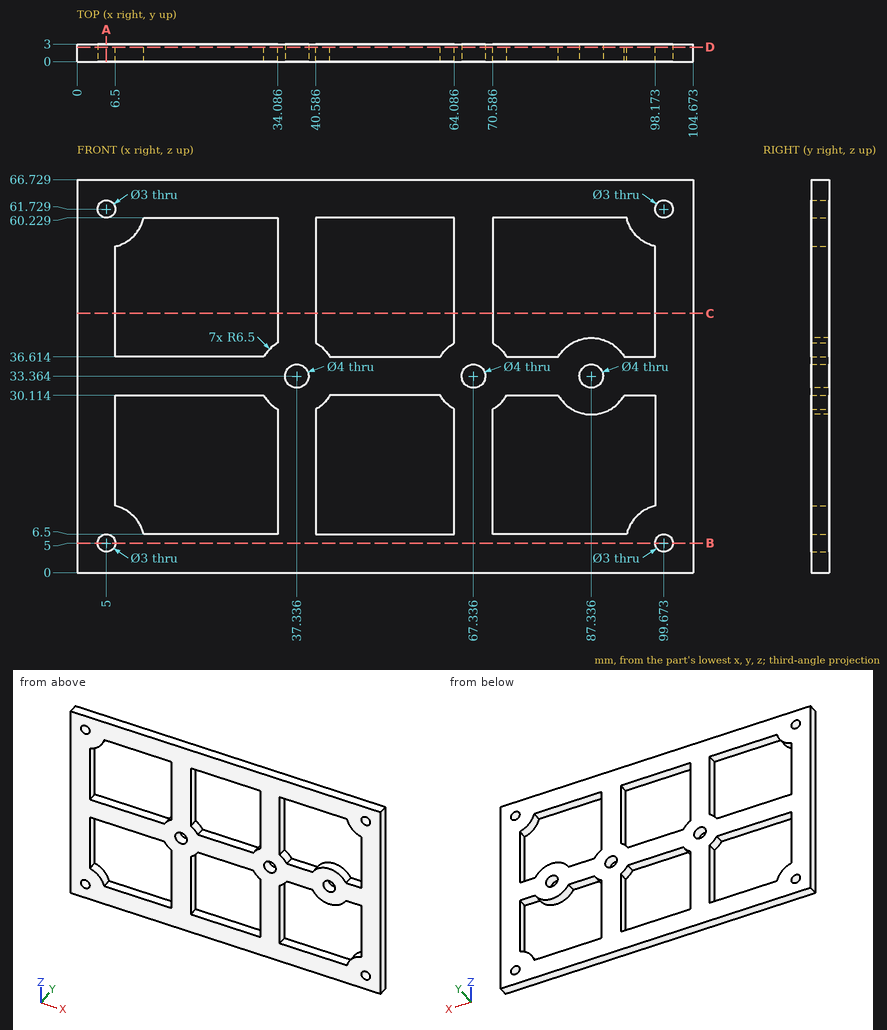
Geometry check sheet. Reference: drawing and pictorial views, mm from the part's lowest x, y, z. Round coordinates to 2 decimals unless told otherwise and drop trailing zeros. Loops run counter-clockwise (first coordinate to the right, second up) from the corner with the lowest first, then second, coordinate; pieces in that order, holes last. Notation, with made-up numbers: (-25.75, -22.75) - (24.25, -22.75) arc R23 cw to (24.25, 15.25) - close; hole circle Ø5 at (64, 61). An arc over 180 degrees is marked (long way). Use a Markdown table: item, result. Add a question column.
1. Section check B-B, the plane z = 5. Record the boundary of the cut face in (x, y).
2. Section check D-D, the plane y = 2.45. Give the number of separate pieces and of enclosed holes in the cut face, plus the area to 3 significant figures.
3. Section check A-A, the plane x = 5. Record the boundary of the cut face in (y, z), plus the area to 3 significant figures.
4. Thickness scan on probe 1 along Z at (x, y) = (80.5, 0.55) (1 decimal); probe 2 along X at (y, z) = (1.75, 54); probe 3 along X at (y, z) = (2, 5). Record the ranges inside material, lowest first. Write a range as [from, to].
5. Section check C-C, the plane z = 44. Record the boundary of the cut face in (x, y).
6. Gauge pin test, flat end, axial feed: pin 1 (3 mm diameter, centred on x = 87.34, z = 33.36, fed in from -Y). Record the tip position at first contact, or that the pin passes through.
Checks:
| question | item | result |
|---|---|---|
| 1 | outline | (0, 0) - (3.5, 0) - (3.5, 3) - (0, 3) - close; (6.5, 0) - (98.17, 0) - (98.17, 3) - (6.5, 3) - close; (101.17, 0) - (104.67, 0) - (104.67, 3) - (101.17, 3) - close |
| 2 | separate pieces | 1 |
| 2 | enclosed holes | 13 |
| 2 | area | 3,350 mm^2 |
| 3 | outline | (0, 0) - (3, 0) - (3, 3.5) - (0, 3.5) - close; (0, 6.5) - (3, 6.5) - (3, 60.23) - (0, 60.23) - close; (0, 63.23) - (3, 63.23) - (3, 66.73) - (0, 66.73) - close |
| 3 | area | 182 mm^2 |
| 4 | probe 1 | z = [0, 6.5], [30.1, 36.6], [60.2, 66.7] |
| 4 | probe 2 | x = [0, 6.5], [34.09, 40.59], [64.09, 70.59], [98.17, 104.67] |
| 4 | probe 3 | x = [0, 3.5], [6.5, 98.17], [101.17, 104.67] |
| 5 | outline | (0, 0) - (6.5, 0) - (6.5, 3) - (0, 3) - close; (34.09, 0) - (40.59, 0) - (40.59, 3) - (34.09, 3) - close; (64.09, 0) - (70.59, 0) - (70.59, 3) - (64.09, 3) - close; (98.17, 0) - (104.67, 0) - (104.67, 3) - (98.17, 3) - close |
| 6 | pin 1 | passes through |
